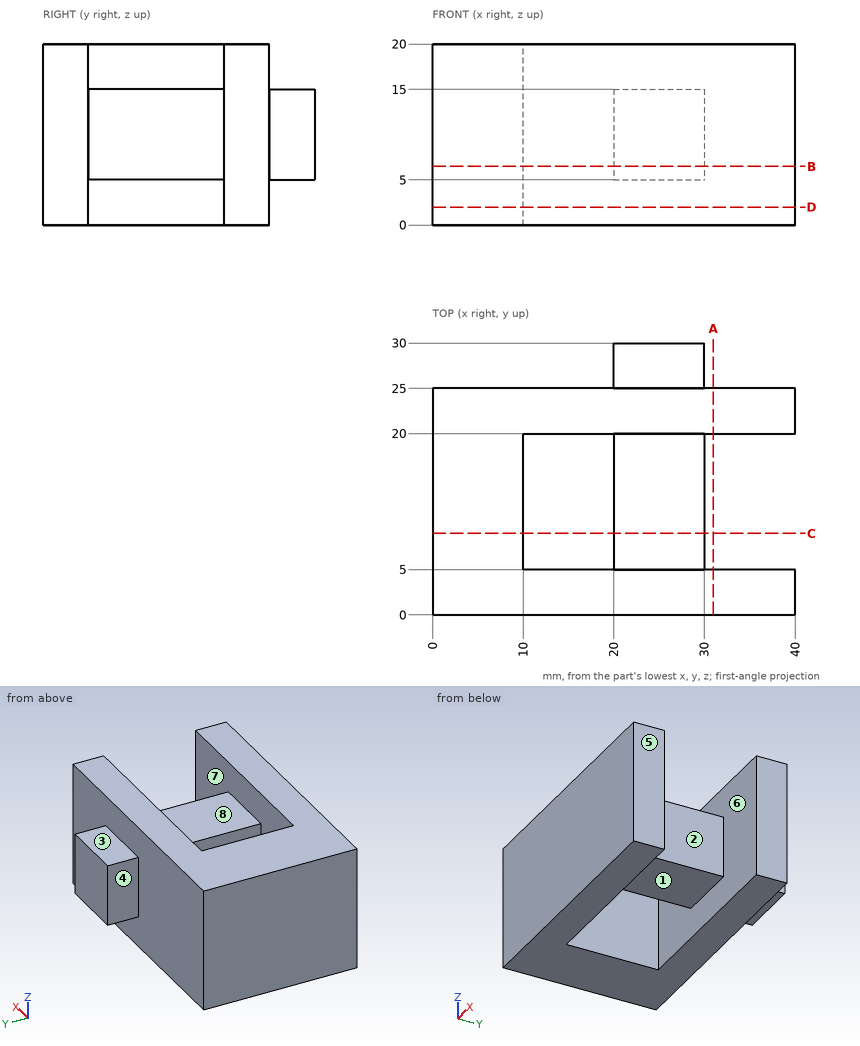
Input: dimensioned drawing with shaded views. Units: mm. Origin: part minimum x, y, z. A direction names the side the tool comes from. Give positions to 0.01 mm unless a question says otherwise; leave off trailing zeros. Order: outer loops, then holes, each group sorted by start corner. A loop starts at its lowest first (then second) coordinate and runs counter-clockwise, first axis right, second up. Notation, with made-up numbers: (-31, 47.25) -> (-13, 47.25) arc R28 cw to (-13, 77.25) -> close; hole circle Ø1 at (2.25, 17). An arc over 180 degrees is marked (long way). Use one line per item in the form item = value.
1) Line query: probe 1 along X at (y, z) = (12.5, 7); probe 2 along Y at (x, z) = (25.5, 17.25); probe 3 along X at (y, z) = (13, 4.5). Output: solid intervals per line, ascending.
Response values:
probe_1 = 0 to 10, 20 to 30
probe_2 = 0 to 5, 20 to 25
probe_3 = 0 to 10
2) Section A-A, the plane x = 31. Return loops of the section in (y, z), and give its area (3 significant figures).
Response values:
outline = (0, 0) -> (5, 0) -> (5, 20) -> (0, 20) -> close; (20, 0) -> (25, 0) -> (25, 20) -> (20, 20) -> close
area = 200 mm^2
3) Section B-B, the plane z = 6.5. Return loops of the section in (x, y), and give its area (3 significant figures).
Response values:
outline = (0, 0) -> (40, 0) -> (40, 5) -> (30, 5) -> (30, 20) -> (40, 20) -> (40, 25) -> (30, 25) -> (30, 30) -> (20, 30) -> (20, 25) -> (0, 25) -> close; hole (10, 5) -> (20, 5) -> (20, 20) -> (10, 20) -> close
area = 750 mm^2
4) Mould query, pull axis X, two halves, no side actions, for the marked faces 5, 6, 7 and 8. Classes: pulls with the +X half, pulls with the -X half, needs draft (parallel to the pull), parting line crosses it, or undercut.
Response values:
face_5 = pulls with the +X half
face_6 = undercut
face_7 = undercut
face_8 = needs draft
5) First-contact query: pin 1 Ø11 at (x, y) = (26, 14) entering from -Z; pin 2 Ø5 at (x, y) = (24, 16) entering from +Z; pin 3 Ø3 at (y, z) = (12.5, 10) entering from +X. Flat tips, straight axial feed; report the tip coordinate or a pass-through.
Response values:
pin_1 = 5
pin_2 = 15
pin_3 = 30
6) Section C-C, the plane y = 9. Return loops of the section in (x, z).
Response values:
outline = (0, 0) -> (10, 0) -> (10, 20) -> (0, 20) -> close; (20, 5) -> (30, 5) -> (30, 15) -> (20, 15) -> close
7) Reachability of the marked faces 1, 2, 3 and 4 from +Z, -Z, +X, -X, +Y, -Y: full face, straight path, thin tool, end or side. Return the list, or none.
Response values:
face_1 = -Z, +X
face_2 = +Z, -Z, +X
face_3 = +Z, +X, -X, +Y
face_4 = +Z, -Z, -X, +Y
8) Section D-D, the plane z = 2. Return loops of the section in (x, y), and give its area (3 significant figures).
Response values:
outline = (0, 0) -> (40, 0) -> (40, 5) -> (10, 5) -> (10, 20) -> (40, 20) -> (40, 25) -> (0, 25) -> close
area = 550 mm^2
